from build123d import *

# Parameters (mm, degrees)
BOSS_EXTRUDE1_DEPTH     = 5
SKETCH3_W               = 139
SKETCH3_H               = 5
BOSS_EXTRUDE2_DEPTH     = 20.4
SKETCH4_W               = 139
SKETCH4_H               = 20.4
BOSS_EXTRUDE3_DEPTH     = 20.5
CUT_EXTRUDE1_DEPTH      = 144.584156508
CUT_EXTRUDE1_DEPTH_BACK = 144.584156508
SKETCH7_W               = 8
SKETCH7_H               = 20.4
CUT_EXTRUDE2_DEPTH      = 20.5
SKETCH8_R               = 2
CUT_EXTRUDE3_DEPTH      = 10


with BuildPart() as part:
    # Sketch1 → Boss-Extrude1 (new body)
    with BuildSketch(Plane(origin=(0, 0, 0), x_dir=(1, 0, 0), z_dir=(0, 1, 0))):
        with BuildLine():
            Line((0, 15.75), (0, 7.75))
            Line((0, 7.75), (6, 7.75))
            ThreePointArc((6, 7.75), (8, 9.75), (10, 7.75))
            Line((10, 7.75), (30, 7.75))
            ThreePointArc((30, 7.75), (32, 9.75), (34, 7.75))
            Line((34, 7.75), (105, 7.75))
            ThreePointArc((105, 7.75), (107, 9.75), (109, 7.75))
            Line((109, 7.75), (129, 7.75))
            ThreePointArc((129, 7.75), (131, 9.75), (133, 7.75))
            Line((133, 7.75), (139, 7.75))
            Line((139, 7.75), (139, 15.75))
            Line((139, 15.75), (133, 15.75))
            ThreePointArc((133, 15.75), (131, 13.75), (129, 15.75))
            Line((129, 15.75), (109, 15.75))
            ThreePointArc((109, 15.75), (107, 13.75), (105, 15.75))
            Line((105, 15.75), (34, 15.75))
            ThreePointArc((34, 15.75), (32, 13.75), (30, 15.75))
            Line((30, 15.75), (24, 15.75))
            Line((24, 15.75), (16, 15.75))
            Line((16, 15.75), (10, 15.75))
            ThreePointArc((10, 15.75), (8, 13.75), (6, 15.75))
            Line((6, 15.75), (0, 15.75))
        make_face()
        with BuildLine():
            Line((0, 7.75), (0, 0))
            Line((0, 0), (139, 0))
            Line((139, 0), (139, 7.75))
            Line((139, 7.75), (133, 7.75))
            ThreePointArc((133, 7.75), (131, 5.75), (129, 7.75))
            Line((129, 7.75), (109, 7.75))
            ThreePointArc((109, 7.75), (107, 5.75), (105, 7.75))
            Line((105, 7.75), (34, 7.75))
            ThreePointArc((34, 7.75), (32, 5.75), (30, 7.75))
            Line((30, 7.75), (10, 7.75))
            ThreePointArc((10, 7.75), (8, 5.75), (6, 7.75))
            Line((6, 7.75), (0, 7.75))
        make_face()
        with BuildLine():
            Line((0, 20.4), (0, 15.75))
            Line((0, 15.75), (6, 15.75))
            ThreePointArc((6, 15.75), (8, 17.75), (10, 15.75))
            Line((10, 15.75), (16, 15.75))
            Line((16, 15.75), (24, 15.75))
            Line((24, 15.75), (30, 15.75))
            ThreePointArc((30, 15.75), (32, 17.75), (34, 15.75))
            Line((34, 15.75), (105, 15.75))
            ThreePointArc((105, 15.75), (107, 17.75), (109, 15.75))
            Line((109, 15.75), (129, 15.75))
            ThreePointArc((129, 15.75), (131, 17.75), (133, 15.75))
            Line((133, 15.75), (139, 15.75))
            Line((139, 15.75), (139, 20.4))
            Line((139, 20.4), (0, 20.4))
        make_face()
        Polygon((0, 23.75), (0, 20.4), (139, 20.4), (139, 25.4), (0, 25.4), align=None)
    extrude(amount=BOSS_EXTRUDE1_DEPTH)

    # Sketch3 → Boss-Extrude2 (add)
    with BuildSketch(Plane(origin=(0, 5, 0), x_dir=(1, 0, 0), z_dir=(0, 1, 0))):
        with Locations((69.5, 22.9)):
            Rectangle(SKETCH3_W, SKETCH3_H)
    extrude(amount=BOSS_EXTRUDE2_DEPTH)

    # Sketch4 → Boss-Extrude3 (add)
    with BuildSketch(Plane(origin=(0, 5, 0), x_dir=(1, 0, 0), z_dir=(0, 1, 0))):
        with Locations((69.5, 10.2)):
            Rectangle(SKETCH4_W, SKETCH4_H)
    extrude(amount=BOSS_EXTRUDE3_DEPTH)

    # Sketch5 → Cut-Extrude1 (cut, two sides: drawn at the far end of the back side and taken through both)
    with BuildSketch(Plane(origin=(139, 0, 0), x_dir=(0, 0, -1), z_dir=(1, 0, 0)).offset(-CUT_EXTRUDE1_DEPTH_BACK)):
        Polygon((0, 5), (20.4, 25.4), (20.4, 25.5), (0, 25.5), align=None)
    extrude(amount=CUT_EXTRUDE1_DEPTH + CUT_EXTRUDE1_DEPTH_BACK, mode=Mode.SUBTRACT)

    # Sketch7 → Cut-Extrude2 (cut)
    with BuildSketch(Plane.XY):
        with Locations((8, 15.2)):
            Rectangle(SKETCH7_W, SKETCH7_H)
        with Locations((32, 15.2)):
            Rectangle(SKETCH7_W, SKETCH7_H)
        with Locations((107, 15.2)):
            Rectangle(SKETCH7_W, SKETCH7_H)
        with Locations((131, 15.2)):
            Rectangle(SKETCH7_W, SKETCH7_H)
    extrude(amount=-CUT_EXTRUDE2_DEPTH, mode=Mode.SUBTRACT)

    # Sketch8 → Cut-Extrude3 (cut)
    with BuildSketch(Plane.XY.offset(-20.5)):
        with Locations((8, 17.4)):
            Circle(SKETCH8_R)
        with Locations((32, 17.4)):
            Circle(SKETCH8_R)
        with Locations((107, 17.4)):
            Circle(SKETCH8_R)
        with Locations((131, 17.4)):
            Circle(SKETCH8_R)
    extrude(amount=-CUT_EXTRUDE3_DEPTH, mode=Mode.SUBTRACT)


solid = part.part
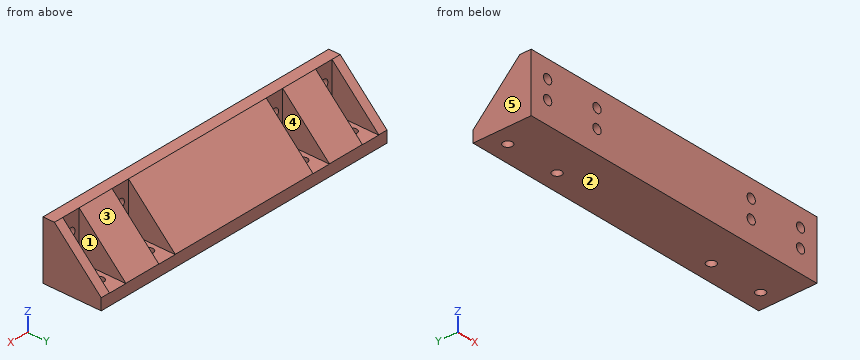
Source: CAD feature listing. Evaluate the final solid. Frame: model axes, mm. Face numbers are marked on the shaded views. A direction names the side the tool comes from. Round coordinates to 2 decimals unless told otherwise and drop trailing zeros. Loops run counter-clockwise (first coordinate to the right, second up) from the corner with the lowest first, then second, coordinate; pieces in that order, holes last. Notation, with made-up numbers: M -19.75,34.25 L -11.75,34.25 A25 cw -11.75,73.25 Z; hole C 25.25,80 d4. An arc over 180 degrees is marked long. Return JSON: item names as keys, results as strings. Group by question number.
1. Section query A-A on z = -1.75. Output: boundary loops of the cut face in (x, y).
2. Pin query (flat end, axial travel): pin 1 (6.5 mm diameter, centred on x = 107, z = -8.5, fed in from +Y); pin 2 (6 mm diameter, centred on x = 45, y = 10, fed in from +Z); pin 3 (4 mm diameter, centred on x = 53.5, z = -5, fed in from +Y). Return the tip coordinate at first contact, or that it passes through.
3. Mould query, pull axis X, two halves, no side actions, for the marked faces 3, 4 and 5. Classes: released by +X, released by -X, zero draft, split by the parting line, or undercut.
4. Section query B-B on x = 32. Output: boundary loops of the cut face in (y, z), and give its area (3 significant figures).
5. Section query C-C on y = 24. Output: boundary loops of the cut face in (x, z).
6. Material intervals for line 1 along X through (y, z) = (11.75, -17.25); line 2 along Z through (x, y) = (8, 2.9); line 3 along X through (y, z) = (3, -6.75), sorted ascending. Write a range as from..to.
7. Section query D-D on z = -15.75. State how many separate pieces and enclosed holes the cut face has, and give its area (3 significant figures).
8. Reachability of the marked faces 1 and 2 from +Z, -Z, +X, -X, +Y, -Y: full face, straight path, thin tool, end or side. Return the list, or none.
Checks:
{
 "1": {"outline": "M 0,0 L 139,0 L 139,6.75 L 135,6.75 L 135,5 L 127,5 L 127,6.75 L 111,6.75 L 111,5 L 103,5 L 103,6.75 L 36,6.75 L 36,5 L 28,5 L 28,6.75 L 12,6.75 L 12,5 L 4,5 L 4,6.75 L 0,6.75 Z"},
 "2": {"pin 1": "stops at y = 5", "pin 2": "stops at z = -2", "pin 3": "stops at y = 12"},
 "3": {"face 3": "zero draft", "face 4": "undercut", "face 5": "released by -X"},
 "4": {"outline": "M 0,-25.4 L 15.4,-25.4 L 15.4,-20.5 L 5,-20.5 L 5,-17.75 L 0,-17.75 Z; M 0,-13.75 L 5,-13.75 L 5,-9.75 L 0,-9.75 Z; M 0,-5.75 L 5,-5.75 L 5,0 L 0,0 Z; M 19.4,-25.4 L 25.4,-25.4 L 25.4,-20.5 L 19.4,-20.5 Z", "area": "167 mm²"},
 "5": {"outline": "M 0,-25.4 L 139,-25.4 L 139,-19 L 135,-19 L 135,-20.5 L 127,-20.5 L 127,-19 L 111,-19 L 111,-20.5 L 103,-20.5 L 103,-19 L 36,-19 L 36,-20.5 L 28,-20.5 L 28,-19 L 12,-19 L 12,-20.5 L 4,-20.5 L 4,-19 L 0,-19 Z"},
 "6": {"line 1": "x = 0..4, 12..28, 36..103, 111..127, 135..139", "line 2": "z = -25.4..-17.75, -13.75..-9.75, -5.75..0", "line 3": "x = 0..6.27, 9.73..30.27, 33.73..105.27, 108.73..129.27, 132.73..139"},
 "7": {"separate pieces": "5", "enclosed holes": "0", "area": "2,300 mm²"},
 "8": {"face 1": "+Z, +Y", "face 2": "-Z, +X, -X, +Y, -Y"}
}
